Geometry check sheet. Reference: the model listing, model coordinates, mm. A direction names the side the tool comes from. Coordinates: 2 decimals unless noted, no trailing zeros. Loops run counter-clockwise (first coordinate to the right, second up) from the corner with the lowest first, then second, coordinate; pieces in that order, holes last. Notation, with made-up numbers: (-4, 74.25) - (20, 74.25) arc R6 cw to (20, 78.25) - close; hole circle Ø2 at (60, 2.25). An arc over 180 degrees is marked (long way). One line per item, written item: value.
from build123d import *

# Parameters (mm, degrees)
SKETCH10_R              = 10
BOSS_EXTRUDE1_DEPTH     = 5
CUT_EXTRUDE3_DEPTH      = 45
CUT_EXTRUDE3_DEPTH_BACK = 20
CUT_EXTRUDE5_DEPTH      = 5
BOSS_EXTRUDE2_DEPTH     = 5
SKETCH14_R              = 1
BOSS_EXTRUDE3_DEPTH     = 3
BOSS_EXTRUDE4_START     = 3
SKETCH15_R              = 1
BOSS_EXTRUDE4_DEPTH     = 3


with BuildPart() as part:
    # Sketch1 → Revolve1 (revolve)
    with BuildSketch(Plane.XY, mode=Mode.PRIVATE) as revolve1_sk:
        with BuildLine():
            Line((20.9, 0), (23.871591838, 0))
            Line((23.871591838, 0), (23.871591838, 4))
            Line((23.871591838, 4), (22.9, 4.236662843))
            Line((22.9, 4.236662843), (22.9, 11.874576818))
            ThreePointArc((22.9, 11.874576818), (23.83692213, 16.100759435), (26.472123903, 19.535021249))
            Line((26.472123903, 19.535021249), (26.427876097, 19.497892931))
            ThreePointArc((26.427876097, 19.497892931), (29.06307787, 22.932154745), (30, 27.158337362))
            Line((30, 27.158337362), (30, 50))
            ThreePointArc((30, 50), (28.828427125, 52.828427125), (26, 54))
            Line((26, 54), (0, 54))
            Line((0, 54), (0, 15))
            Line((0, 15), (19.9, 15))
            ThreePointArc((19.9, 15), (20.607106781, 14.707106781), (20.9, 14))
            Line((20.9, 14), (20.9, 0))
        make_face()
    revolve(revolve1_sk.sketch.rotate(Axis((0, 0, 0), (0, 1, 0)), 90), axis=Axis((0, 0, 0), (0, 1, 0)))

    # Sketch10 → Boss-Extrude1 (add)
    with BuildSketch(Plane(origin=(0, 0, -30), x_dir=(-1, 0, 0), z_dir=(0, 0, -1))):
        with Locations((3.346345887, 38.658337362)):
            Circle(SKETCH10_R)
    extrude(amount=-BOSS_EXTRUDE1_DEPTH)

    # Sketch11 → Cut-Extrude3 (cut, two sides: drawn at the far end of the back side and taken through both)
    with BuildSketch(Plane(origin=(0, 17, 0), x_dir=(1, 0, 0), z_dir=(0, 1, 0)).offset(-CUT_EXTRUDE3_DEPTH_BACK)):
        with BuildLine():
            Line((-14.735085045, 0), (20.264914955, 0))
            ThreePointArc((20.264914955, 0), (2.764914955, 17.5), (-14.735085045, 0))
        make_face()
    extrude(amount=CUT_EXTRUDE3_DEPTH + CUT_EXTRUDE3_DEPTH_BACK, mode=Mode.SUBTRACT)

    # Sketch9 → Cut-Extrude5 (cut)
    with BuildSketch(Plane(origin=(0, 54, 0), x_dir=(1, 0, 0), z_dir=(0, 1, 0))):
        with BuildLine():
            Line((-30, 0), (30, 0))
            ThreePointArc((30, 0), (0, 30), (-30, 0))
        make_face()
    extrude(amount=-CUT_EXTRUDE5_DEPTH, mode=Mode.SUBTRACT)

    # Sketch13 → Boss-Extrude2 (add)
    with BuildSketch(Plane(origin=(0, 0, 0), x_dir=(-1, 0, 0), z_dir=(0, 0, -1))):
        with BuildLine():
            Line((22.5, 53.5), (26.5, 53.5))
            ThreePointArc((26.5, 53.5), (26.853553391, 53.353553391), (27, 53))
            Line((27, 53), (27, 51))
            ThreePointArc((27, 51), (26.853553391, 50.646446609), (26.5, 50.5))
            Line((26.5, 50.5), (22.5, 50.5))
            ThreePointArc((22.5, 50.5), (22.146446609, 50.646446609), (22, 51))
            Line((22, 51), (22, 53))
            ThreePointArc((22, 53), (22.146446609, 53.353553391), (22.5, 53.5))
        make_face()
        with BuildLine():
            Line((-26.5, 53.5), (-22.5, 53.5))
            ThreePointArc((-22.5, 53.5), (-22.146446609, 53.353553391), (-22, 53))
            Line((-22, 53), (-22, 51))
            ThreePointArc((-22, 51), (-22.146446609, 50.646446609), (-22.5, 50.5))
            Line((-22.5, 50.5), (-26.5, 50.5))
            ThreePointArc((-26.5, 50.5), (-26.853553391, 50.646446609), (-27, 51))
            Line((-27, 51), (-27, 53))
            ThreePointArc((-27, 53), (-26.853553391, 53.353553391), (-26.5, 53.5))
        make_face()
    extrude(amount=BOSS_EXTRUDE2_DEPTH)

    # Sketch14 → Boss-Extrude3 (add)
    with BuildSketch(Plane.ZY.offset(-22)):
        with Locations(Location((-3, 52, 0), (0, 0, 270))):
            Circle(SKETCH14_R)
    extrude(amount=BOSS_EXTRUDE3_DEPTH)

    # Sketch15 → Boss-Extrude4 (add)
    with BuildSketch(Plane(origin=(-22, 0, 0), x_dir=(0, 0, -1), z_dir=(1, 0, 0)).offset(BOSS_EXTRUDE4_START)):
        with Locations(Location((3, 52, 0), (0, 0, 270))):
            Circle(SKETCH15_R)
    extrude(amount=-BOSS_EXTRUDE4_DEPTH)


solid = part.part
(1) Material ranges on probe 1 along X at (y, z) = (3.5, 0); probe 2 along X at (y, z) = (11.25, 0); probe 3 along Y at (x, z) = (7, 17), recorded low to high. Write a range as from..to.
Reply:
probe 1: -23.87..-20.9, 20.9..23.87
probe 2: -22.9..-20.9, 20.9..22.9
probe 3: 15..54
(2) Access from +Z, -Z, +X, -X, +Y, -Y to the whole of each face (thin tool, end or side, straight path). Record for faces 5 (the face through (-23.67, 2.03, 3.11)), 6 (the face through (-22, 52, -4.4)), 7 (the face through (19, 52, -3)), 8 (the face through (27, 52, -2)), 9 (the face through (-27, 52, -2)).
Reply:
face 5: -Y
face 6: -Z
face 7: -Z, +Y, -Y
face 8: -Z, +X, +Y
face 9: -Z, -X, +Y
(3) Cross-section at B-B on y = 32.5. Record the cut outline in (x, z), and give its area (3 significant figures).
Reply:
outline: (-11.23, -30) - (4.53, -30) - (4.53, -29.66) arc R30 ccw (long way) to (-11.23, -27.82) - close; hole (-14.74, 0) arc R17.5 ccw to (20.26, 0) - close
area: 2,350 mm2
(4) Release check for a two-part mould opening along Y. For faces 1 (the face through (22.355, 8.109, 4.964)), 2 (the face through (0, 54, 10)), 3 (the face through (24, 52, -5)), 4 (the face through (-20.479, 52.737, -3.676)) record: pulls with the +Y half, pulls with the -Y half, needs draft (parallel to the pull), parting line crosses it, or undercut.
Reply:
face 1: undercut
face 2: pulls with the +Y half
face 3: needs draft
face 4: undercut
(5) Cross-section at A-A on y = 52. Record the cut outline in (x, z), and give its area (3 significant figures).
Reply:
outline: (-29.46, 0) - (-27, 0) - (-27, -5) - (-22, -5) - (-22, -4) - (-19, -4) - (-19, -2) - (-22, -2) - (-22, 0) - (22, 0) - (22, -2) - (19, -2) - (19, -4) - (22, -4) - (22, -5) - (27, -5) - (27, 0) - (29.46, 0) arc R29.46 ccw to start
area: 1,430 mm2
(6) Go/stop test with flat-tipped pins: pin 1 Ø1 at (y, z) = (52, -4.5) entering from +X; pin 2 Ø6 at (y, z) = (16.5, -12.5) entering from -X; pin 3 Ø4 at (x, y) = (19, 20.5) entering from +Z; pin 4 Ø4.5 at (x, z) = (-24, -2.5) entering from -Y. Record where each tip stops, or that it passes through.
Reply:
pin 1: x = 27
pin 2: x = -23.58
pin 3: z = 22.45
pin 4: y = 0
